Input: part model. Units: mm. Frame: model coordinates. A direction names the side the tool comes from. Give positions to 0.01 mm unless a question says otherwise; leave off trailing zeros. Loops run counter-clockwise (first coordinate to the right, second up) from the corner with the lowest first, then second, coordinate; pieces in that order, holes last.
from build123d import *

# Parameters (mm, degrees)
F0_W     = 10.16
F0_H     = 25.4
F0_W_2   = 6.604
F0_H_2   = 15.24
F1_DEPTH = 19.97964
F2_R     = 5.07999


# Not quite as in the source:
# - a fillet or chamfer is up to 0.001 mm smaller than in the source, because OpenCascade refuses the exact size


with BuildPart() as f1:
    # F0 (on Right) → F1 (new body)
    with BuildSketch(Plane.YZ):
        with Locations((6.7968953631, 12.7)):
            Rectangle(F0_W, F0_H)
        with Locations((6.7968953631, 12.7)):
            Rectangle(F0_W_2, F0_H_2, mode=Mode.SUBTRACT)
    extrude(amount=F1_DEPTH)

    # F2 (radius 5.08 in the source; OpenCascade refuses exactly that, so slightly less here)
    f2_edges = [f1.edges().sort_by_distance(p)[0] for p in [
        (9.98982, 1.716895, 25.4),
        (9.98982, 11.876895, 25.4),
        (9.98982, 1.716895, 0),
        (9.98982, 11.876895, 0),
    ]]
    fillet(f2_edges, radius=F2_R)


solid = f1.part
(1) Mould query, pull axis Y, two halves, no side actions, for faces 3 (the cylindrical face through (10.1, 10.3, 1.4)), 4 (the flat face through (0, 3, 13)), 5 (the flat face through (10, 3.495, 13)), 6 (the flat face through (10, 1.717, 13)). Classes: +Y half, -Y half, draft (parallel to the pull), parting line (faces both ways), or undercut.
Values follow:
face 3: +Y half
face 4: draft
face 5: undercut
face 6: -Y half
(2) Ray query, probe 1 along Y at (x, z) = (2.75, 5.5); probe 2 along Y at (x, z) = (1.5, 5); probe 3 along Z at (x, y) = (14.25, 4.75). Return the intervals inside material, ascending.
Values follow:
probe 1: y = 1.72 to 3.49, 10.1 to 11.88
probe 2: y = 1.72 to 11.88
probe 3: z = 0.43 to 5.08, 20.32 to 24.97
(3) Cut plane A-A (z = 14). Return the cut outline in (x, y), and give its area (3 significant figures).
Values follow:
outline: (0, 1.72) - (19.98, 1.72) - (19.98, 3.49) - (0, 3.49) - close; (0, 10.1) - (19.98, 10.1) - (19.98, 11.88) - (0, 11.88) - close
area: 71.0 mm2
(4) Reachability of faces 1 (the flat face through (10, 7, 20.32)), 2 (the cylindrical face through (10.13, 3.166, 1.528)) from +Z, -Z, +X, -X, +Y, -Y: full face, straight path, thin tool, end or side. Return the list, or none.
Values follow:
face 1: +X, -X
face 2: -Z, +X, -X, -Y
(5) Cut plane B-B (y = 9.5). Return the cut outline in (x, z), and give its area (3 significant figures).
Values follow:
outline: (0, 0.78) - (19.98, 0.78) - (19.98, 5.08) - (0, 5.08) - close; (0, 20.32) - (19.98, 20.32) - (19.98, 24.62) - (0, 24.62) - close
area: 172 mm2
(6) Cut plane D-D (y = 2.5). Return the cut outline in (x, z).
Values follow:
outline: (0, 2.37) - (19.98, 2.37) - (19.98, 23.03) - (0, 23.03) - close
